Could you check a few things on this drawing? It's one solid part, dimensions in mm from its lowest x, y, z. A direction names the side the tool comes from. Round coordinates to 2 decimals unless told otherwise and drop trailing zeros. Loops run counter-clockwise (first coordinate to the right, second up) from the corner with the lowest first, then second, coordinate; pieces in that order, holes last. Notation, with made-up numbers: (10.5, -1) -> (36.5, -1) arc R11 ccw to (36.5, 14) -> close; hole circle Ø8 at (-23.75, 89.25). An arc over 180 degrees is marked (long way). Use CSV: the item, a comma, the result in double quotes. Start each with the question number.
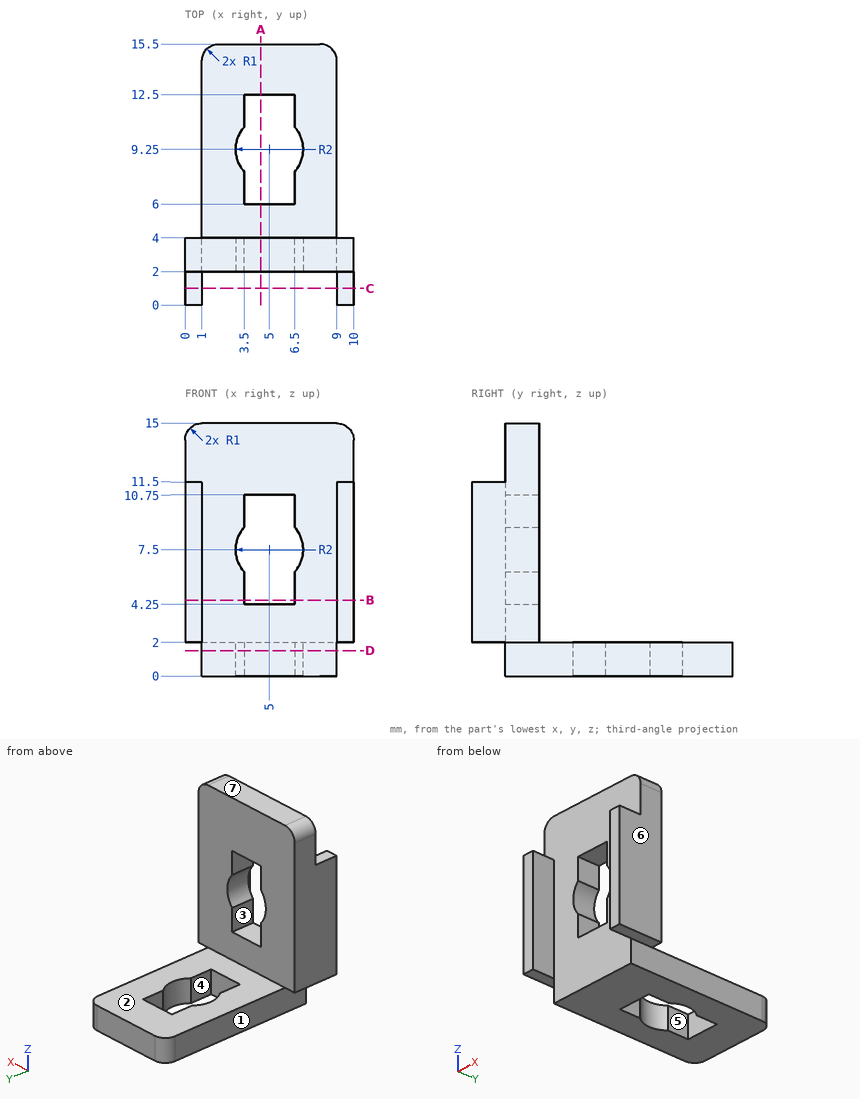
Q1. I want a section at A-A, the plane x = 4.5. List the corners of the cut face in (y, z) for me.
Q2. I want a section at B-B, the plane z = 4.5. List the corners of the cut face in (x, y) for me, then the cut area to 3 significant figures.
Q3. For the marked faces 1, 2, 3 and 4, which set-ups out of +Z, -Z, +X, -X, +Y, -Y let a thin tool reach every point of the face, with its end or its side?
Q4. I need wall thicknesses on line 1 along X through (y, z) = (3.75, 9.25); line 2 along Z through (x, y) = (8, 14.25); line 3 along X through (y, z) = (7, 1.5). Which ranges of each line are inside material? Lowest first, please.
Q5. Will these pins go through, and if not, where does the flat tip stop? pin 1 Ø1.5 at (y, z) = (7, 1) entering from +X; pin 2 Ø2 at (y, z) = (11.5, 1.5) entering from -X; pin 3 Ø0.8 at (x, y) = (0.5, 1) entering from +Z.
Q6. I want a section at C-C, the plane y = 1. List the corners of the cut face in (x, z) for me.
Q7. If we mould it in two halves opening along X, with no side actions, what happens to the marked faces 5, 6 and 7? For each: pulls with the +X half, pulls with the -X half, needs draft (parallel to the pull), parting line crosses it, or undercut.
Q8. I want a section at D-D, the plane z = 1.5. List the corners of the cut face in (x, y) for me, then the cut area to 3 significant figures.
Values found:
1,outline,"(2, 0) -> (6, 0) -> (6, 2) -> (4, 2) -> (4, 4.25) -> (2, 4.25) -> close; (2, 10.75) -> (4, 10.75) -> (4, 15) -> (2, 15) -> close; (12.5, 0) -> (15.5, 0) -> (15.5, 2) -> (12.5, 2) -> close"
2,outline,"(0, 0) -> (1, 0) -> (1, 2) -> (3.5, 2) -> (3.5, 4) -> (0, 4) -> close; (6.5, 2) -> (9, 2) -> (9, 0) -> (10, 0) -> (10, 4) -> (6.5, 4) -> close"
2,area,"18.0 mm2"
3,face 1,"-Z, -X, +Y, -Y"
3,face 2,"+Z, +X, -X, +Y"
3,face 3,"+Y, -Y"
3,face 4,"+Z, -Z"
4,line 1,"0 to 3.5, 6.5 to 10"
4,line 2,"0 to 2"
4,line 3,"1 to 3.5, 6.5 to 9"
5,pin 1,"x = 9"
5,pin 2,"x = 1"
5,pin 3,"z = 11.5"
6,outline,"(0, 2) -> (1, 2) -> (1, 11.5) -> (0, 11.5) -> close; (9, 2) -> (10, 2) -> (10, 11.5) -> (9, 11.5) -> close"
7,face 5,"undercut"
7,face 6,"pulls with the +X half"
7,face 7,"needs draft"
8,outline,"(1, 2) -> (9, 2) -> (9, 14.5) arc R1 ccw to (8, 15.5) -> (2, 15.5) arc R1 ccw to (1, 14.5) -> close; hole (3.5, 6) -> (6.5, 6) -> (6.5, 7.93) arc R2 ccw to (6.5, 10.57) -> (6.5, 12.5) -> (3.5, 12.5) -> (3.5, 10.57) arc R2 ccw to (3.5, 7.93) -> close"
8,area,"86.3 mm2"
